```python
from build123d import *

# Parameters (mm, degrees)
SKETCH2_R                      = 2.5000000000000027
BOSS_EXTRUDE2_DEPTH            = 5
SKETCH3_R                      = 3.750000000000007
SKETCH3_R_2                    = 2.5000000000000027
SKETCH3_R_3                    = 3.7500000000000036
SKETCH3_R_4                    = 3.7500000000000138
SKETCH3_R_5                    = 3.7499999999999916
BOSS_EXTRUDE3_DEPTH            = 3
FILLET1_R                      = 3.75
BOSS_EXTRUDE4_DEPTH            = 5
CBORE_FOR_M3_SHCS1_D           = 3.4
CBORE_FOR_M3_SHCS1_CBORE_D     = 6.2
CBORE_FOR_M3_SHCS1_CBORE_DEPTH = 3
SKETCH8_R                      = 2.5000000000000027
BOSS_EXTRUDE5_DEPTH            = 4
FILLET2_R                      = 2


with BuildPart() as part:
    # Sketch2 → Boss-Extrude2 (new body)
    with BuildSketch(Plane(origin=(0, 0, 0), x_dir=(1, 0, 0), z_dir=(0, 1, 0))):
        Polygon((45.660000000000004, 40.58000000000002), (-45.65999999999999, 40.58000000000002), (-45.65999999999999, -40.580000000000005), (-38.24999999999999, -40.580000000000005), (-38.25000000000001, -48.07999999999986), (-38.25000000000001, -86.82999999999993), (38.25000000000002, -86.82999999999993), (38.25000000000001, -48.0799999999999), (38.25000000000002, -40.57999999999999), (45.660000000000004, -40.57999999999999), align=None)
        with Locations(Location((-41.90999999999999, 36.83000000000001, 0), (0, 0, 270))):
            Circle(SKETCH2_R, mode=Mode.SUBTRACT)
        with Locations(Location((41.910000000000004, 36.83000000000001, 0), (0, 0, 270))):
            Circle(SKETCH2_R, mode=Mode.SUBTRACT)
        with Locations(Location((-41.90999999999999, -36.82999999999999, 0), (0, 0, 270))):
            Circle(SKETCH2_R, mode=Mode.SUBTRACT)
        with Locations(Location((41.910000000000004, -36.82999999999999, 0), (0, 0, 270))):
            Circle(SKETCH2_R, mode=Mode.SUBTRACT)
        with Locations(Location((-34.50000000000001, -48.07999999999986, 0), (0, 0, 270))):
            Circle(SKETCH2_R, mode=Mode.SUBTRACT)
        with Locations(Location((-34.49999999999999, -83.0799999999999, 0), (0, 0, 270))):
            Circle(SKETCH2_R, mode=Mode.SUBTRACT)
        with Locations(Location((34.49999999999999, -83.0799999999999, 0), (0, 0, 270))):
            Circle(SKETCH2_R, mode=Mode.SUBTRACT)
        with Locations(Location((34.50000000000001, -48.0799999999999, 0), (0, 0, 270))):
            Circle(SKETCH2_R, mode=Mode.SUBTRACT)
        Polygon((38.16, -28.542299400797987), (5.680831716333313, 2.429e-14), (38.16, 28.542299400798022), align=None, mode=Mode.SUBTRACT)
        Polygon((-38.15999999999998, -28.54229940079798), (-38.15999999999999, 28.54229940079801), (-5.680831716333299, 1.041e-14), align=None, mode=Mode.SUBTRACT)
        Polygon((31.96192690435635, 33.08000000000001), (6.94e-15, 4.992246053747464), (-31.96192690435633, 33.08000000000001), align=None, mode=Mode.SUBTRACT)
        Polygon((31.96192690435635, -33.079999999999984), (7.81e-15, -4.992246053747436), (-31.961926904356336, -33.079999999999984), align=None, mode=Mode.SUBTRACT)
        Polygon((-30.749999999999986, -44.32999999999987), (-3.75, -44.32999999999987), (-3.749999999999986, -40.58), (-30.74999999999999, -40.580000000000005), align=None, mode=Mode.SUBTRACT)
        Polygon((30.75, -81.57832850736624), (30.750000000000004, -54.18702415953998), (3.7500000000000004, -67.88267633345322), align=None, mode=Mode.SUBTRACT)
        Polygon((30.750000000000004, -44.32999999999987), (30.750000000000018, -40.57999999999999), (3.7500000000000138, -40.58), (3.750000000000019, -44.32999999999987), align=None, mode=Mode.SUBTRACT)
        Polygon((-27.896704771665014, -83.9353526669063), (27.896704771665014, -83.9353526669063), (0, -69.78485024649659), align=None, mode=Mode.SUBTRACT)
        Polygon((-27.896704771665025, -51.82999999999982), (-2.8e-16, -65.98050242040974), (27.896704771665025, -51.82999999999982), align=None, mode=Mode.SUBTRACT)
        Polygon((-30.750000000000004, -54.18702415953998), (-3.749999999999999, -67.88267633345322), (-30.75, -81.57832850736624), align=None, mode=Mode.SUBTRACT)
    extrude(amount=BOSS_EXTRUDE2_DEPTH)

    # Sketch3 → Boss-Extrude3 (add)
    # profile 1 of 8: a face of its own
    with BuildSketch(Plane(origin=(0, 5, 0), x_dir=(1, 0, 0), z_dir=(0, 1, 0))):
        with Locations(Location((-41.90999999999999, 36.83000000000001, 0), (0, 0, 90))):
            Circle(SKETCH3_R)
        with Locations(Location((-41.90999999999999, 36.83000000000001, 0), (0, 0, 270))):
            Circle(SKETCH3_R_2, mode=Mode.SUBTRACT)
    # profile 2 of 8: a face of its own
    with BuildSketch(Plane(origin=(0, 5, 0), x_dir=(1, 0, 0), z_dir=(0, 1, 0))):
        with Locations(Location((41.910000000000004, 36.83000000000001, 0), (0, 0, 90))):
            Circle(SKETCH3_R)
        with Locations(Location((41.910000000000004, 36.83000000000001, 0), (0, 0, 270))):
            Circle(SKETCH3_R_2, mode=Mode.SUBTRACT)
    # profile 3 of 8: a face of its own
    with BuildSketch(Plane(origin=(0, 5, 0), x_dir=(1, 0, 0), z_dir=(0, 1, 0))):
        with Locations(Location((41.910000000000004, -36.82999999999999, 0), (0, 0, 270))):
            Circle(SKETCH3_R)
        with Locations(Location((41.910000000000004, -36.82999999999999, 0), (0, 0, 270))):
            Circle(SKETCH3_R_2, mode=Mode.SUBTRACT)
    # profile 4 of 8: a face of its own
    with BuildSketch(Plane(origin=(0, 5, 0), x_dir=(1, 0, 0), z_dir=(0, 1, 0))):
        with Locations(Location((-41.90999999999999, -36.82999999999999, 0), (0, 0, 270))):
            Circle(SKETCH3_R)
        with Locations(Location((-41.90999999999999, -36.82999999999999, 0), (0, 0, 270))):
            Circle(SKETCH3_R_2, mode=Mode.SUBTRACT)
    # profile 5 of 8: a face of its own
    with BuildSketch(Plane(origin=(0, 5, 0), x_dir=(1, 0, 0), z_dir=(0, 1, 0))):
        with Locations(Location((-34.50000000000001, -48.07999999999986, 0), (0, 0, 180))):
            Circle(SKETCH3_R_3)
        with Locations(Location((-34.50000000000001, -48.07999999999986, 0), (0, 0, 270))):
            Circle(SKETCH3_R_2, mode=Mode.SUBTRACT)
    # profile 6 of 8: a face of its own
    with BuildSketch(Plane(origin=(0, 5, 0), x_dir=(1, 0, 0), z_dir=(0, 1, 0))):
        with Locations(Location((-34.49999999999999, -83.0799999999999, 0), (0, 0, 270))):
            Circle(SKETCH3_R_3)
        with Locations(Location((-34.49999999999999, -83.0799999999999, 0), (0, 0, 270))):
            Circle(SKETCH3_R_2, mode=Mode.SUBTRACT)
    # profile 7 of 8: a face of its own
    with BuildSketch(Plane(origin=(0, 5, 0), x_dir=(1, 0, 0), z_dir=(0, 1, 0))):
        with Locations(Location((34.49999999999999, -83.0799999999999, 0), (0, 0, 270))):
            Circle(SKETCH3_R_4)
        with Locations(Location((34.49999999999999, -83.0799999999999, 0), (0, 0, 270))):
            Circle(SKETCH3_R_2, mode=Mode.SUBTRACT)
    # profile 8 of 8: a face of its own
    with BuildSketch(Plane(origin=(0, 5, 0), x_dir=(1, 0, 0), z_dir=(0, 1, 0))):
        with Locations((34.50000000000001, -48.0799999999999)):
            Circle(SKETCH3_R_5)
        with Locations(Location((34.50000000000001, -48.0799999999999, 0), (0, 0, 270))):
            Circle(SKETCH3_R_2, mode=Mode.SUBTRACT)
    extrude(amount=BOSS_EXTRUDE3_DEPTH)

    # Fillet1
    fillet1_edges = [part.edges().sort_by_distance(p)[0] for p in [
        (-45.65999999999999, 2.5, -40.58000000000002),
        (38.25000000000002, 2.5, 86.82999999999993),
        (-38.25000000000001, 2.5, 86.82999999999993),
        (-45.65999999999999, 2.5, 40.580000000000005),
        (45.660000000000004, 2.5, 40.57999999999999),
        (45.660000000000004, 2.5, -40.58000000000002),
    ]]
    fillet(fillet1_edges, radius=FILLET1_R)

    # Sketch4 → Boss-Extrude4 (add)
    with BuildSketch(Plane.XZ):
        Polygon((-45.65999999999999, -19.975), (-55.66, -19.975), (-55.66, -9.975000000000001), (-45.65999999999999, -9.975000000000003), align=None)
        Polygon((45.660000000000004, -19.975), (55.66000000000001, -19.975), (55.660000000000004, -9.974999999999998), (45.660000000000004, -9.975000000000001), align=None)
        Polygon((-38.25000000000007, 56.224999999999994), (-48.25000000000008, 56.225), (-48.25000000000008, 66.22500000000001), (-38.25000000000007, 66.22500000000001), align=None)
        Polygon((38.25000000000002, 66.22500000000001), (48.250000000000014, 66.22500000000001), (48.25000000000002, 56.224999999999994), (38.25000000000002, 56.224999999999994), align=None)
    extrude(amount=-BOSS_EXTRUDE4_DEPTH)

    # CBORE for M3 SHCS1 (through all)
    with Locations(Plane(origin=(0, 5, 0), x_dir=(1, 0, 0), z_dir=(0, 1, 0))):
        with Locations((50.66, 14.975), (-50.66, 14.975), (-43.25, -61.225), (43.25, -61.225)):
            CounterBoreHole(CBORE_FOR_M3_SHCS1_D / 2, CBORE_FOR_M3_SHCS1_CBORE_D / 2, CBORE_FOR_M3_SHCS1_CBORE_DEPTH)

    # Sketch8 → Boss-Extrude5 (add)
    with BuildSketch(Plane.XZ):
        with Locations(Location((-34.49999999999999, 83.0799999999999, 0), (0, 0, 270))):
            Circle(SKETCH8_R)
        with Locations(Location((34.49999999999999, 83.0799999999999, 0), (0, 0, 270))):
            Circle(SKETCH8_R)
        with Locations(Location((34.50000000000001, 48.0799999999999, 0), (0, 0, 270))):
            Circle(SKETCH8_R)
        with Locations(Location((41.910000000000004, 36.82999999999999, 0), (0, 0, 270))):
            Circle(SKETCH8_R)
        with Locations(Location((41.910000000000004, -36.83000000000001, 0), (0, 0, 270))):
            Circle(SKETCH8_R)
        with Locations(Location((-41.90999999999999, -36.83000000000001, 0), (0, 0, 270))):
            Circle(SKETCH8_R)
        with Locations(Location((-41.90999999999999, 36.82999999999999, 0), (0, 0, 270))):
            Circle(SKETCH8_R)
        with Locations(Location((-34.50000000000001, 48.07999999999986, 0), (0, 0, 270))):
            Circle(SKETCH8_R)
    extrude(amount=-BOSS_EXTRUDE5_DEPTH)

    # Fillet2
    fillet2_edges = [part.edges().sort_by_distance(p)[0] for p in [
        (27.896704771665025, 2.5, 51.82999999999982),
        (-27.896704771665025, 2.5, 51.82999999999982),
        (-27.896704771665014, 2.5, 83.9353526669063),
        (27.896704771665014, 2.5, 83.9353526669063),
        (-30.750000000000004, 2.5, 54.18702415953998),
        (-30.75, 2.5, 81.57832850736624),
        (-31.961926904356336, 2.5, 33.079999999999984),
        (31.96192690435635, 2.5, 33.079999999999984),
        (31.96192690435635, 2.5, -33.08000000000001),
        (-31.96192690435633, 2.5, -33.08000000000001),
        (-38.15999999999999, 2.5, -28.54229940079801),
        (-38.15999999999998, 2.5, 28.54229940079798),
        (38.16, 2.5, -28.542299400798022),
        (38.16, 2.5, 28.542299400797987),
        (30.75, 2.5, 81.57832850736624),
        (30.750000000000004, 2.5, 54.18702415953998),
    ]]
    fillet(fillet2_edges, radius=FILLET2_R)


solid = part.part
```
For this review, take the finished solid that the model builds, in its own axes (mm). A direction names the side the tool comes from. Round coordinates to 2 decimals unless told otherwise and drop trailing zeros. Write each loop counter-clockwise with the first axis right and the second up, starting at its lowest first coordinate (ties: lowest second). Pieces come first, ordered by that corner, then holes. Notation, with made-up numbers: (-16, 18) - (1, 18) arc R18 cw to (1, 43) - close; hole circle Ø1 at (59.5, 49.25). An arc over 180 degrees is marked (long way). Write each question's results on one line, items separated by ' | '.
Item 1: Take a section at B-B on z = -31. State the section outline as (x, y) points.
Calculated:
outline: (-45.66, 0) - (-28.65, 0) - (-28.65, 5) - (-45.66, 5) - close; (28.65, 0) - (45.66, 0) - (45.66, 5) - (28.65, 5) - close
Item 2: Take a section at A-A on x = -50.66. State the section outline as (y, z) points (3 decimals).
Calculated:
outline: (0, -19.975) - (5, -19.975) - (5, -18.075) - (2, -18.075) - (2, -16.675) - (0, -16.675) - close; (0, -13.275) - (2, -13.275) - (2, -11.875) - (5, -11.875) - (5, -9.975) - (0, -9.975) - close
Item 3: Draft analysis for pull direction X (two halves, no side actions). For faces 1 (the face through (10.36, 2.46, 75.04)), 2 (the face through (-38.25, 2, 75)), 3 (the face through (-39, 8, -38)), state which applies: pulls with the +X half, pulls with the -X half, needs draft (parallel to the pull), parting line crosses it, or undercut.
Calculated:
face 1: undercut | face 2: pulls with the -X half | face 3: needs draft
Item 4: For faces 4 (the face through (43, 2, 66.225)), 5 (the face through (21.486, 2.535, 82.364)), 6 (the face through (34.012, 6.479, 44.362)), 7 (the face through (0, 2, 86.83)), 8 (the face through (32, 8, 84)), list the 3-axis set-ups (+Z, -Z, +X, -X, +Y, -Y) from which the entire face can be reached by the end or side of a thin tool; tool diameter is ignored.
Calculated:
face 4: +Z, +X, +Y, -Y | face 5: +Y, -Y | face 6: +Y | face 7: +Z, +X, -X, +Y, -Y | face 8: +Z, -Z, +X, -X, +Y
Item 5: To check wall thickness, follow line 1 along X through (y, z) = (2.5, 43.5); line 2 along X through (y, z) = (3, 68.5); line 3 along Z through (x, y) = (-50.66, 1.55) (3 decimals). State the ranges of each line that lie inside material, in increasing order. Write a range as from..to.
Calculated:
line 1: x = -38.25..-30.75, -3.75..3.75, 30.75..38.25 | line 2: x = -38.25..-30.75, -4.97..4.97, 30.75..38.25 | line 3: z = -19.975..-16.675, -13.275..-9.975
Item 6: For pin 1 (1.1 mm diameter, centred on y = 3.5, z = 42.5, fed in from -X); pin 2 (4 mm diameter, centred on y = 2.5, z = 61.5, fed in from -X); pin 3 (2.5 mm diameter, centred on x = 42, z = 38, fed in from +Y), all flat-tipped, find the tip position at first contact; note any pin that passes through.
Calculated:
pin 1: stops at x = -38.25 | pin 2: stops at x = -48.25 | pin 3: stops at y = 4
